```python
from build123d import *

# Parameters (mm, degrees)
BOSS_EXTRUDE1_DEPTH = 100
SKETCH4_R           = 20
BOSS_EXTRUDE3_DEPTH = 38
BOSS_EXTRUDE4_DEPTH = 10
FILLET1_R           = 10
FILLET2_R           = 5
BOSS_EXTRUDE5_DEPTH = 6
FILLET3_R           = 20
BOSS_EXTRUDE6_DEPTH = 6
HOLE1_D             = 12
HOLE1_DEPTH         = 44


with BuildPart() as part:
    # Sketch1 → Boss-Extrude1 (new body)
    with BuildSketch(Plane(origin=(0, 0, 0), x_dir=(0, 0, -1), z_dir=(1, 0, 0))):
        Polygon((20, -136), (44, -136), (44, -150), (0, -150), (0, 150), (44, 150), (44, 136), (20, 136), align=None)
    extrude(amount=BOSS_EXTRUDE1_DEPTH)



with BuildPart() as body_2:
    # Sketch4 → Boss-Extrude3 (new, symmetric)
    with BuildSketch(Plane(origin=(50, 0, 0), x_dir=(0, 0, -1), z_dir=(1, 0, 0))):
        with BuildLine():
            Line((-269, 119), (-269, 68))
            Line((-269, 68), (-280, 68))
            Line((-280, 68), (-280, 95.314561435))
            ThreePointArc((-280, 95.314561435), (-328.115831839, 132.057564857), (-269, 119))
        make_face()
        with Locations((-300, 119)):
            Circle(SKETCH4_R, mode=Mode.SUBTRACT)
    extrude(amount=BOSS_EXTRUDE3_DEPTH, both=True)


with BuildPart() as part_1:
    add(part.part)

    add(body_2.part)  # Boss-Extrude4 merges body 2
    # Sketch7 → Boss-Extrude4 (add)
    with BuildSketch(Plane.XZ.offset(-68)):
        Polygon((88, 280), (12, 280), (12, 269), (0, 0), (0, -5), (100, -5), (100, 0), (88, 269), align=None)
    extrude(amount=-BOSS_EXTRUDE4_DEPTH)

    # Fillet1
    fillet1_edges = [part_1.edges().sort_by_distance(p)[0] for p in [
        (50, 68, 280),
        (50, 78, 269),
    ]]
    fillet(fillet1_edges, radius=FILLET1_R)

    # Fillet2
    fillet2_edges = [part_1.edges().sort_by_distance(p)[0] for p in [
        (50, 95.314561435, 280),
    ]]
    fillet(fillet2_edges, radius=FILLET2_R)

    # Sketch8 → Boss-Extrude5 (add, symmetric)
    with BuildSketch(Plane(origin=(50, 0, 0), x_dir=(0, 0, -1), z_dir=(1, 0, 0))):
        with BuildLine():
            Line((0, 78), (-70, 78))
            ThreePointArc((-70, 78), (-20.502525317, 98.502525317), (0, 148))
            Line((0, 148), (0, 78))
        make_face()
    extrude(amount=BOSS_EXTRUDE5_DEPTH, both=True)

    # Fillet3
    fillet3_edges = [part_1.edges().sort_by_distance(p)[0] for p in [
        (78, 78, 0),
        (50, 68, 0),
        (22, 78, 0),
    ]]
    fillet(fillet3_edges, radius=FILLET3_R)

    # Sketch10 → Boss-Extrude6 (add, symmetric)
    with BuildSketch(Plane(origin=(50, 0, 0), x_dir=(0, 0, -1), z_dir=(1, 0, 0))):
        with BuildLine():
            Line((-331, 119), (-331, 40))
            ThreePointArc((-331, 40), (-310.497474683, -9.497474683), (-261, -30))
            Line((-261, -30), (-70, -30))
            ThreePointArc((-70, -30), (-20.502525317, -50.502525317), (0, -100))
            Line((0, -100), (0, 48))
            ThreePointArc((0, 48), (-5.857864376, 62.142135624), (-20, 68))
            Line((-20, 68), (-269, 68))
            Line((-269, 68), (-270, 68))
            ThreePointArc((-270, 68), (-277.071067812, 70.928932188), (-280, 78))
            Line((-280, 78), (-280, 86.273863656))
            ThreePointArc((-280, 86.273863656), (-282.299691376, 90.481990714), (-287.083333333, 90.819160371))
            ThreePointArc((-287.083333333, 90.819160371), (-316.741913471, 92.909612243), (-331, 119))
        make_face()
    extrude(amount=BOSS_EXTRUDE6_DEPTH, both=True)

    # Hole1
    with Locations(Plane.XY):
        with Locations((50, -118), (22, 128), (78, 128)):
            Hole(HOLE1_D / 2, depth=HOLE1_DEPTH)


solid = part_1.part
```
Geometry check sheet. Reference: the model listing, model coordinates, mm. A direction names the side the tool comes from. Give positions to 0.01 mm unless a question says otherwise; leave off trailing zeros. Order: outer loops, then holes, each group sorted by start corner. A loop starts at its lowest first (then second) coordinate and runs counter-clockwise, first axis right, second up.
1. Access from +Z, -Z, +X, -X, +Y, -Y to the whole of each face (thin tool, end or side, straight path). Record for faces 1 (the face through (50.54, 80.85, 265.99)), 2 (the face through (88, 100, 286)), 3 (the face through (72, 82, 280)), 4 (the face through (56, 92, 17)), 5 (the face through (49, 2, -20)).
2. Gauge pin test, flat ends, axial feed: pin 1 Ø3 at (x, z) = (84, 35.5) entering from +Y; pin 2 Ø3.5 at (x, z) = (48, 148) entering from -Y; pin 3 Ø12 at (x, y) = (40.5, -102.5) entering from -Z. Record the tip position at first contact, or that the pin passes through.
3. Section check C-C, the plane z = 300. Enter the section's corners in (x, y).
4. Thickness scan on L1, parallel to Y at x = 22, z = -11; L2, parallel to Y at x = 44.5, z = -26; L3, parallel to Z at x = 82.5, y = -35. Record the ranges inside material, lowest first.
5. Section check B-B, the plane y = -118. Enter the section's corners in (x, z).
6. Section check A-A, the plane x = 50. Enter the section's corners in (y, z).
7. Section check D-D, the plane x = 32.5. Enter the section's corners in (y, z).
8. Release check for a two-part mould opening along Y. For faces 6 (the face through (27.78, 70.85, 276.99)), 7 (the face through (22.308, 83.703, 6.014)), 8 (the face through (49, 143, -44)), 9 (the face through (49, -136, -32)) record: pulls with the +Y half, pulls with the -Y half, needs draft (parallel to the pull), parting line crosses it, or undercut.
Values follow:
1. face 1: +X, -X, +Y
1. face 2: +Z, +X, +Y, -Y
1. face 3: +Z, +X, -Y
1. face 4: +X, +Y
1. face 5: -Z, +X, -X
2. pin 1: stops at y = 78
2. pin 2: stops at y = -30
2. pin 3: stops at z = -20
3. outline: (12, 88) - (44, 88) - (44, -18.13) - (56, -18.13) - (56, 88) - (88, 88) - (88, 99) - (12, 99) - close; (12, 139) - (88, 139) - (88, 150) - (12, 150) - close
4. L1: y = -150 to 122, 134 to 150
4. L2: y = -150 to -136, 136 to 150
4. L3: z = -20 to 0
5. outline: (0, -20) - (44, -20) - (44, 0) - (0, 0) - close; (56, -20) - (100, -20) - (100, 0) - (56, 0) - close
6. outline: (-150, -44) - (-136, -44) - (-136, -20) - (-124, -20) - (-124, 0) - (-150, 0) - close; (-112, -20) - (136, -20) - (136, -44) - (150, -44) - (150, 0) - (148, 0) arc R70 cw to (78, 70) - (78, 259) arc R10 cw to (88, 269) - (119, 269) arc R31 ccw to (119, 331) - (40, 331) arc R70 ccw to (-30, 261) - (-30, 70) arc R70 cw to (-100, 0) - (-112, 0) - close; hole circle Ø40 at (119, 300)
7. outline: (-150, -44) - (-136, -44) - (-136, -20) - (136, -20) - (136, -44) - (150, -44) - (150, 0) - (98, 0) arc R20 cw to (78, 20) - (78, 259) arc R10 cw to (88, 269) - (119, 269) arc R31 ccw (long way) to (90.82, 287.08) arc R5 cw to (86.27, 280) - (78, 280) arc R10 ccw to (68, 270) - (68, 20) arc R20 cw to (48, 0) - (-150, 0) - close; hole circle Ø40 at (119, 300)
8. face 6: pulls with the -Y half
8. face 7: pulls with the +Y half
8. face 8: needs draft
8. face 9: undercut
